Verification items for the finished model (mm, model axes). Face numbers are marked on the shaded views. Coordinates: 2 decimals unless noted, no trailing zeros. Write item = value, one per line. Start each with the question number.
1. Release check for a two-part mould opening along Y. For the marked faces 1 and 2 record: +Y half, -Y half, draft (parallel to the pull), parting line (faces both ways), or undercut.
2. Thickness scan on line 1 along Z through (x, y) = (0, 10). Record the ranges inside material, lowest first. Write a range as from..to.
3. Go/stop test with a flat-tipped pin: P1, Ø1.5, axis at x = -3, z = 0, coming from the -Y side. Record where the tip stops, or that it passes through.
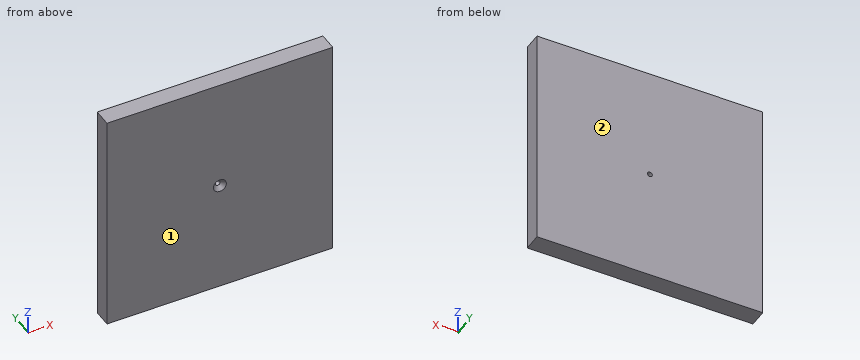
Autodesk Inventor part; units mm, degrees
ref_plane "YZ Plane" through (0, 0, 0) normal (1, 0, 0) x (0, 1, 0)
ref_plane "XZ Plane" through (0, 0, 0) normal (0, 1, 0) x (-1, 0, 0)
ref_plane "XY Plane" through (0, 0, 0) normal (0, 0, 1) x (1, 0, 0)
sketch "Sketch1" plane through (0, 0, 0) normal (0, 1, 0) x (-1, 0, 0)
  line L0 (75, -75) -> (-75, -75)
  line L1 (-75, -75) -> (-75, 75)
  line L2 (-75, 75) -> (75, 75)
  line L3 (75, 75) -> (75, -75)
  point P0 (0, 0)
  point P1 (75, 0)
  point P2 (0, -75)
  dimension "d0" = 150
  dimension "d1" = 150
extrude "Extrusion1" add sketch "Sketch1" along normal blind 12
sketch "Sketch2" plane through (0, 0, 0) normal (0, -1, 0) x (1, 0, 0)
  point P0 (0, 0)
  point P1 (0, 0)
hole "Hole1" at (0, 0, 0) direction (0, 1, 0) diameter 3.242 end through all countersink diameter 8.6 countersink angle 90
properties part number "Camera_base_plate"
Worked out:
q1.face_1 = -Y half
q1.face_2 = +Y half
q2.line_1 = -75..-1.62, 1.62..75
q3.P1 = 0.55
